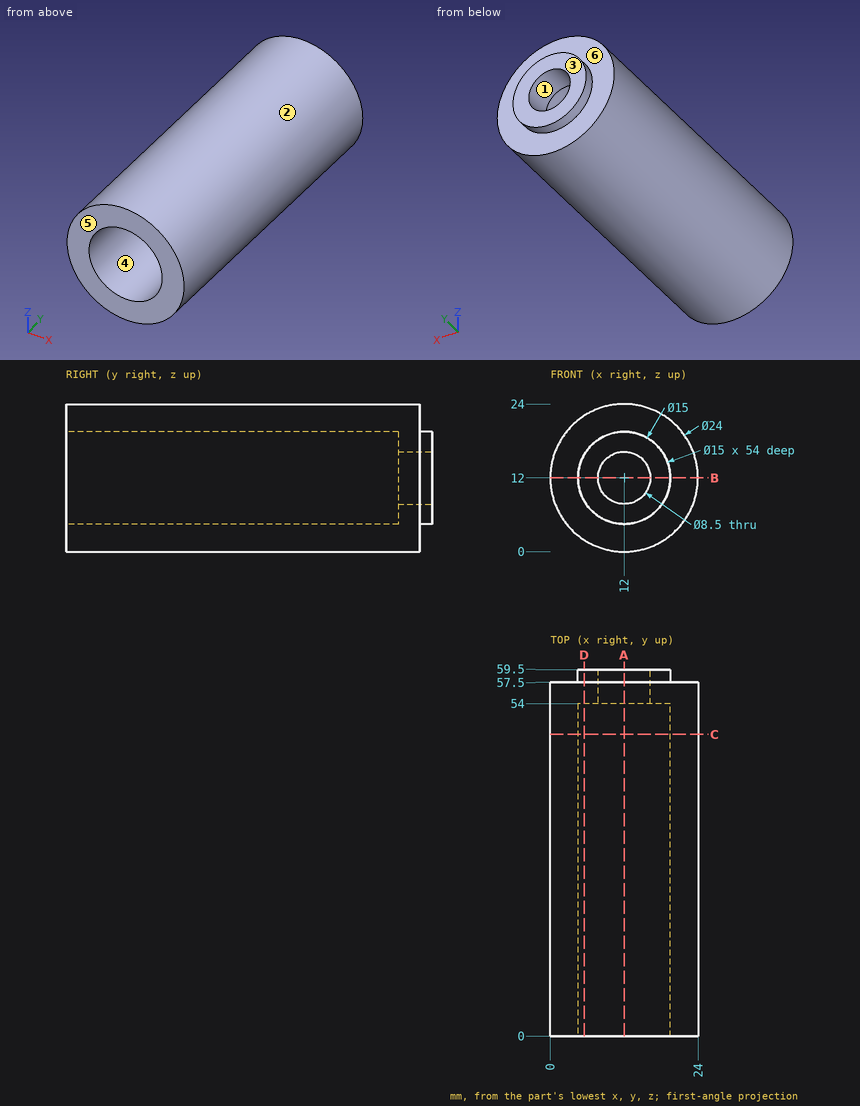
Input: dimensioned drawing with shaded views. Units: mm. Origin: part minimum x, y, z. A direction names the side the tool comes from. Give positions to 0.01 mm unless a question says otherwise; leave off trailing zeros. Write each loop counter-clockwise with the first axis right and the second up, starting at its lowest first coordinate (ties: lowest second). Pieces come first, ordered by that corner, then holes.
Q1. Section A-A, the plane x = 12. Output: boundary loops of the cut face in (y, z).
Q2. Section B-B, the plane z = 12. Output: boundary loops of the cut face in (x, y).
Q3. Material intervals for probe 1 along Z at (x, y) = (12, 19); probe 2 along Y at (x, z) = (11.75, 5); probe 3 along Z at (x, y) = (12, 57.15), sorted ascending.
Q4. First-contact query: P1, Ø5, axis at x = 20, y = 18.5, coming from the +Z side; P2, Ø1.5, axis at x = 8, z = 2.5, coming from the +Y side; P3, Ø10, axis at x = 13.5, z = 11.5, coming from the -Y side. Flat tips, straight axial feed; report the tip coordinate or a pass-through.
Q5. Section D-D, the plane x = 5.5. Output: boundary loops of the cut face in (y, z).
Q6. Pull-direction query (X, two-part tool) for the marked faces 1, 2 and 3; classes: pulls with the +X half, pulls with the -X half, needs draft (parallel to the pull), parting line crosses it, or undercut.
Q7. Set-up query: the marked faces 4, 5 and 6. Return all of +Z, -Z, +X, -X, +Y, -Y with unobstructed straight access to the full face (end or side cutting, diameter ignored); none if empty.
Q8. Section C-C, the plane y = 49. Output: boundary loops of the cut face in (x, z), plus the area to 3 significant figures.
Filled in:
1. outline: (0, 0) - (57.5, 0) - (57.5, 4.5) - (59.5, 4.5) - (59.5, 7.75) - (54, 7.75) - (54, 4.5) - (0, 4.5) - close; (0, 19.5) - (54, 19.5) - (54, 16.25) - (59.5, 16.25) - (59.5, 19.5) - (57.5, 19.5) - (57.5, 24) - (0, 24) - close
2. outline: (0, 0) - (4.5, 0) - (4.5, 54) - (7.75, 54) - (7.75, 59.5) - (4.5, 59.5) - (4.5, 57.5) - (0, 57.5) - close; (16.25, 54) - (19.5, 54) - (19.5, 0) - (24, 0) - (24, 57.5) - (19.5, 57.5) - (19.5, 59.5) - (16.25, 59.5) - close
3. probe 1: z = 0 to 4.5, 19.5 to 24
3. probe 2: y = 54 to 59.5
3. probe 3: z = 0 to 7.75, 16.25 to 24
4. P1: stops at z = 22.67
4. P2: stops at y = 57.5
4. P3: stops at y = 54
5. outline: (0, 1.91) - (57.5, 1.91) - (57.5, 8.26) - (59.5, 8.26) - (59.5, 15.74) - (57.5, 15.74) - (57.5, 22.09) - (0, 22.09) - (0, 15.74) - (54, 15.74) - (54, 8.26) - (0, 8.26) - close
6. face 1: undercut
6. face 2: parting line crosses it
6. face 3: needs draft
7. face 4: -Y
7. face 5: +Z, -Z, +X, -X, -Y
7. face 6: +Y
8. outline: circle Ø24 at (12, 12); hole circle Ø15 at (12, 12)
8. area: 276 mm2
